For this review, use the dimensioned drawing (mm, ordinates from the lowest corner) and the shaded views. Coordinates: 2 decimals unless noted, no trailing zeros. Write each loop counter-clockwise with the first axis right and the second up, starting at its lowest first coordinate (ties: lowest second). Pieces come first, ordered by that corner, then holes. Notation, with made-up numbers: M 47,89 L 85,89 A24 cw 85,117 Z; hole C -5,-33.5 d1. An arc over 180 degrees is marked long. Return JSON: item names as keys, results as strings. Group by question number.
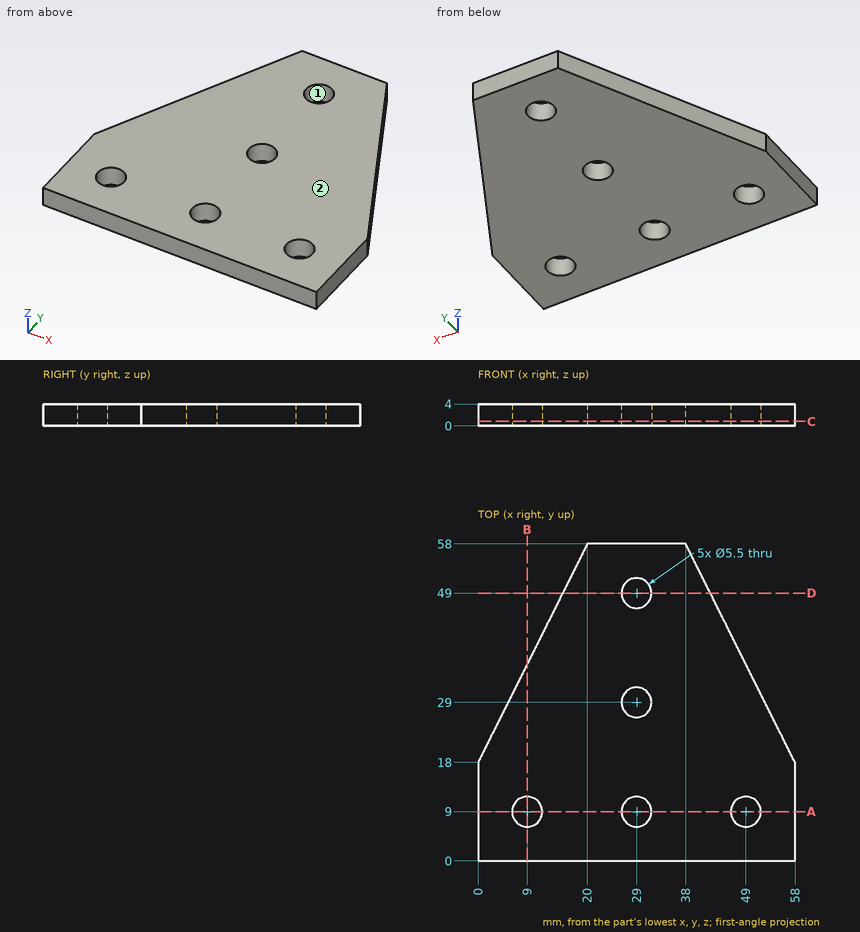
Item 1: For line 1 (Y direction, x = 29, z = 1.8); line 2 (X direction, y = 47.5, z = 1.15); line 3 (X direction, y = 47, z = 2.8), list the stretches that pass through material, from the lowest coordinate up.
Item 2: Add section C-C (z = 0.8). Write out the cut boundary in (x, y).
Item 3: Add section D-D (y = 49). Write out the cut boundary in (x, z).
Item 4: The part is to be moulded in two halves that separate along X. For the marked faces 1 and 2, say which applies: pulls with the +X half, pulls with the -X half, needs draft (parallel to the pull), parting line crosses it, or undercut.
Item 5: Add section B-B (x = 9). Write out the cut boundary in (y, z), plus the area to 3 significant figures.
Item 6: Add section A-A (y = 9). Write out the cut boundary in (x, z).
Geometry check:
{
 "1": {"line 1": "0 to 6.25, 11.75 to 26.25, 31.75 to 46.25, 51.75 to 58", "line 2": "14.75 to 26.7, 31.3 to 43.25", "line 3": "14.5 to 27.11, 30.89 to 43.5"},
 "2": {"outline": "M 0,0 L 58,0 L 58,18 L 38,58 L 20,58 L 0,18 Z; hole C 9,9 d5.5; hole C 29,9 d5.5; hole C 29,29 d5.5; hole C 29,49 d5.5; hole C 49,9 d5.5"},
 "3": {"outline": "M 15.5,0 L 26.25,0 L 26.25,4 L 15.5,4 Z; M 31.75,0 L 42.5,0 L 42.5,4 L 31.75,4 Z"},
 "4": {"face 1": "undercut", "face 2": "needs draft"},
 "5": {"outline": "M 0,0 L 6.25,0 L 6.25,4 L 0,4 Z; M 11.75,0 L 36,0 L 36,4 L 11.75,4 Z", "area": "122 mm^2"},
 "6": {"outline": "M 0,0 L 6.25,0 L 6.25,4 L 0,4 Z; M 11.75,0 L 26.25,0 L 26.25,4 L 11.75,4 Z; M 31.75,0 L 46.25,0 L 46.25,4 L 31.75,4 Z; M 51.75,0 L 58,0 L 58,4 L 51.75,4 Z"}
}
